Could you check a few things on this model? Use its own coordinates, in mm. Face numbers are marked on the shaded views. A direction names the side the tool comes from. Give positions to 0.01 mm unless a question says otherwise; leave off trailing zeros. Write each loop counter-clockwise with the first axis right and the second up, starting at its lowest first coordinate (ties: lowest second). Pieces come first, ordered by that corner, then holes. Notation, with made-up numbers: M 3.25,4.25 L 47.25,4.25 A25 ccw 47.25,21.25 Z; hole C 76,-36 d8. An arc over 180 degrees is marked long. One line per item, written item: value.
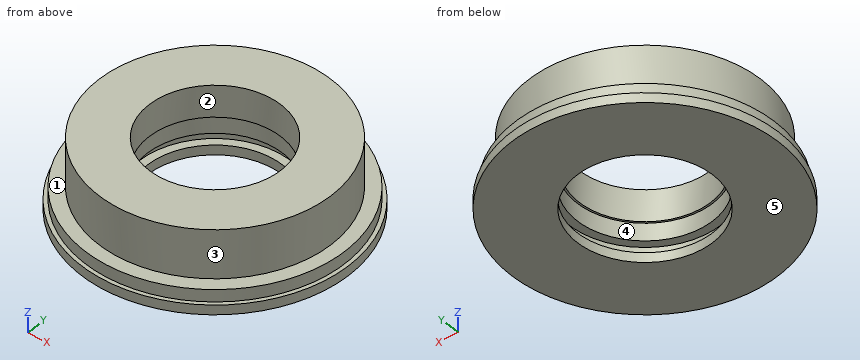
```python
from build123d import *

# Parameters (mm, degrees)
SKETCH1_R           = 70
BOSS_EXTRUDE1_DEPTH = 40
SKETCH3_W           = 14
SKETCH3_H           = 32.4
SKETCH5_W           = 26.233930481
SKETCH5_H           = 6
SKETCH6_W           = 149.593137009
SKETCH6_H           = 50.047703926
CUT_EXTRUDE1_DEPTH  = 86


with BuildPart() as part:
    # Sketch1 → Boss-Extrude1 (new body, symmetric)
    with BuildSketch(Plane.XY):
        Circle(SKETCH1_R)
    extrude(amount=BOSS_EXTRUDE1_DEPTH, both=True)

    # Sketch2 → Cut-Revolve1 (revolve, cut)
    with BuildSketch(Plane(origin=(0, 0, 0), x_dir=(1, 0, 0), z_dir=(0, 1, 0))):
        Polygon((-69, 40), (-69, 35), (-67, 35), (-67, 28.7), (-60, 28.7), (-60, 3.7), (-67, 3.7), (-67, -2.6), (-69, -2.6), (-69, -44.705491592), (-73.643536697, -44.705491592), (-73.643536697, 40), align=None)
    revolve(axis=Axis((0, 0, 0), (0, 0, -1)), mode=Mode.SUBTRACT)

    # Sketch3 → Cut-Revolve2 (revolve, cut)
    with BuildSketch(Plane(origin=(0, 0, 0), x_dir=(1, 0, 0), z_dir=(0, 1, 0))):
        with Locations((-62, -23.8)):
            Rectangle(SKETCH3_W, SKETCH3_H)
    revolve(axis=Axis((0, 0, 0), (0, 0, 1)), mode=Mode.SUBTRACT)

    # Sketch4 → Cut-Revolve3 (revolve, cut)
    with BuildSketch(Plane(origin=(0, 0, 0), x_dir=(1, 0, 0), z_dir=(0, 1, 0))):
        Polygon((0, 42.623044552), (-35, 42.623044552), (-35, 20), (-34, 20), (-34, -40), (0, -40), align=None)
    revolve(axis=Axis((0, 0, 0), (0, 0, -1)), mode=Mode.SUBTRACT)

    # Sketch5 → Cut-Revolve4 (revolve, cut)
    with BuildSketch(Plane(origin=(0, 0, 0), x_dir=(1, 0, 0), z_dir=(0, 1, 0))):
        with Locations((-26.133034759, 32)):
            Rectangle(SKETCH5_W, SKETCH5_H)
    revolve(axis=Axis((0, 0, 0), (0, 0, -1)), mode=Mode.SUBTRACT)

    # Sketch6 → Cut-Extrude1 (cut, symmetric)
    with BuildSketch(Plane(origin=(0, 0, 0), x_dir=(1, 0, 0), z_dir=(0, 1, 0))):
        with Locations((-0.733299692, -21.323851963)):
            Rectangle(SKETCH6_W, SKETCH6_H)
    extrude(amount=CUT_EXTRUDE1_DEPTH, both=True, mode=Mode.SUBTRACT)


solid = part.part
```
1) If we section it at B-B, the plane y = -27.5: Write out the boundary of the cut face in (x, z), then the cut area to 3 significant figures.
Outcome:
outline: M -63.28,-40 L -21.65,-40 L -21.65,-35 L -28.01,-35 L -28.01,-29 L -21.65,-29 L -21.65,-20 L -19.99,-20 L -19.99,-3.7 L -53.33,-3.7 L -53.33,-28.7 L -61.1,-28.7 L -61.1,-35 L -63.28,-35 Z; M 19.99,-20 L 21.65,-20 L 21.65,-29 L 28.01,-29 L 28.01,-35 L 21.65,-35 L 21.65,-40 L 63.28,-40 L 63.28,-35 L 61.1,-35 L 61.1,-28.7 L 53.33,-28.7 L 53.33,-3.7 L 19.99,-3.7 Z
area: 2,470 mm^2
2) Please list where these lines run through material, in increasing order: L1, parallel to Y at x = 0, z = -38.85; L2, parallel to Z at x = -31, y = -18.5; L3, parallel to Z at x = -6, y = 63. Write a range as from..to.
Outcome:
L1: y = -69..-35, 35..69
L2: z = -40..-35, -29..-3.7
L3: z = -40..-28.7
3) I'm going to push flat-ended pins straight in: pin 1 (3 mm diameter, centred on y = 41, z = -28, fed in from -X); pin 2 (8 mm diameter, centred on x = 39.5, z = -13, fed in from +Y); pin 3 (3 mm diameter, centred on y = -24.5, z = -10.5, fed in from -X). Where does each tip first touch, or does it pass through?
Outcome:
pin 1: stops at x = -53.99
pin 2: stops at y = 48.37
pin 3: stops at x = -55.42
4) If we section it at A-A, the plane x = 0: Write out the boundary of the cut face in (y, z).
Outcome:
outline: M -69,-40 L -35,-40 L -35,-35 L -39.25,-35 L -39.25,-29 L -35,-29 L -35,-20 L -34,-20 L -34,-3.7 L -60,-3.7 L -60,-28.7 L -67,-28.7 L -67,-35 L -69,-35 Z; M 34,-20 L 35,-20 L 35,-29 L 39.25,-29 L 39.25,-35 L 35,-35 L 35,-40 L 69,-40 L 69,-35 L 67,-35 L 67,-28.7 L 60,-28.7 L 60,-3.7 L 34,-3.7 Z
5) If we section it at D-D, the plane y = 55.5: Write out the boundary of the cut face in (x, z).
Outcome:
outline: M -41,-40 L 41,-40 L 41,-35 L 37.53,-35 L 37.53,-28.7 L 22.8,-28.7 L 22.8,-3.7 L -22.8,-3.7 L -22.8,-28.7 L -37.53,-28.7 L -37.53,-35 L -41,-35 Z
6) We'd pull the mould along Y, two halves only. Please class the marked faces 3, 4 and 5: pulls with the +Y half, pulls with the -Y half, needs draft (parallel to the pull), parting line crosses it, or undercut.
Outcome:
face 3: parting line crosses it
face 4: undercut
face 5: needs draft
7) If we section it at C-C, the plane z = -12: Write out the boundary of the cut face in (x, y).
Outcome:
outline: C 0,0 d120; hole C 0,0 d68
8) On a 3-axis mill with a long thin cutter (end or side, diameter ignored), from which of +Z, -Z, +X, -X, +Y, -Y can I reach the whole of each face in a straight line? I mean the marked faces 1 and 2. Say none if no direction works.
Outcome:
face 1: +Z
face 2: +Z, -Z
